Input: part model. Units: mm. Frame: model coordinates. A direction names the side the tool comes from. Give positions to 0.01 mm unless a question says otherwise; leave off trailing zeros. Loops run counter-clockwise (first coordinate to the right, second up) from the corner with the lowest first, then second, coordinate; pieces in that order, holes last. Notation, with made-up numbers: (3.25, -32.75) -> (44.25, -32.75) arc R27 cw to (44.25, -1.75) -> close; hole circle Ø7 at (30, -40). An arc over 180 degrees is marked (long way). Use CSV: the item, a comma, the result in double quotes.
```python
from build123d import *

# Parameters (mm, degrees)
BOX044_W                  = 180
BOX044_H                  = 123
BOX044_DEPTH              = 8
BOX045_W                  = 140
BOX045_H                  = 90
BOX045_DEPTH              = 40
CYLINDER019_R             = 15
CYLINDER019_DEPTH         = 10
CYLINDER020_R             = 15
CYLINDER020_DEPTH         = 24
BOX046_W                  = 75
BOX046_H                  = 13
BOX046_DEPTH              = 20
BOX047_W                  = 171
BOX047_H                  = 15
BOX047_DEPTH              = 10
FUSION013_ROLL_ANGLE      = -90
FUSION013_PLACEMENT_ANGLE = -180


with BuildPart() as cube039:
    # Box044 → Box044 (new body)
    with BuildSketch(Plane.XY):
        with Locations((90, 61.5)):
            Rectangle(BOX044_W, BOX044_H)
    extrude(amount=BOX044_DEPTH)


with BuildPart() as cube040:
    # Box045 → Box045 (new body)
    with BuildSketch(Plane(origin=(10, 15, 0), x_dir=(1, 0, 0), z_dir=(0, 0, 1))):
        with Locations((70, 45)):
            Rectangle(BOX045_W, BOX045_H)
    extrude(amount=BOX045_DEPTH)


with BuildPart() as cylinder019:
    # Cylinder019 → Cylinder019 (new body)
    with BuildSketch(Plane(origin=(30, 104, 24), x_dir=(1, 0, 0), z_dir=(0, 1, 0))):
        Circle(CYLINDER019_R)
    extrude(amount=CYLINDER019_DEPTH)


with BuildPart() as cylinder020:
    # Cylinder020 → Cylinder020 (new body)
    with BuildSketch(Plane(origin=(130, 104, 24), x_dir=(1, 0, 0), z_dir=(0, 1, 0))):
        Circle(CYLINDER020_R)
    extrude(amount=CYLINDER020_DEPTH)


with BuildPart() as cube041:
    # Box046 → Box046 (new body)
    with BuildSketch(Plane(origin=(193, 25, 0), x_dir=(0, 1, 0), z_dir=(0, 0, 1))):
        with Locations((37.5, 6.5)):
            Rectangle(BOX046_W, BOX046_H)
    extrude(amount=BOX046_DEPTH)


with BuildPart() as f_120_back:
    # Box047 → Box047 (new body)
    with BuildSketch(Plane(origin=(3, 0, 8), x_dir=(1, 0, 0), z_dir=(0, 0, 1))):
        with Locations((85.5, 7.5)):
            Rectangle(BOX047_W, BOX047_H)
    extrude(amount=BOX047_DEPTH)

    # Fusion013: union Cube039, Cube040, Cylinder019, Cylinder020, Cube041
    add(cube039.part)
    add(cube040.part)
    add(cylinder019.part)
    add(cylinder020.part)
    add(cube041.part)


with BuildPart() as f_120_back_1:
    # Fusion013 roll: moved
    add(f_120_back.part.rotate(Axis((0, 0, 0), (1, 0, 0)), FUSION013_ROLL_ANGLE))


with BuildPart() as f_120_back_2:
    # Fusion013 placement: moved
    add(f_120_back_1.part.moved(Location((195, -80, 185))).rotate(Axis((195, -80, 185), (0, 0, 1)), FUSION013_PLACEMENT_ANGLE))


solid = f_120_back_2.part
```
1) Ray query, line 1 (X direction, y = -95, z = 143); line 2 (X direction, y = -94, z = 177); line 3 (Z direction, x = 65, y = -101). Return the intervals inside material, ascending.
From the geometry:
line 1,"x = 2 to 15, 45 to 185"
line 2,"x = 21 to 192"
line 3,"z = 57 to 170"
2) Contact query for flat-ended pins moving along their axis: pin 1 (14.5 mm diameter, centred on x = 6.5, y = -93.5, fed in from +Z); pin 2 (8 mm diameter, centred on y = -94, z = 177, fed in from +X); pin 3 (15 mm diameter, centred on x = 163, y = -103, fed in from -Z). Output: stop coordinate, or through.
From the geometry:
pin 1,"stops at z = 160"
pin 2,"stops at x = 192"
pin 3,"stops at z = 71"
3) Reachability of faces 4 (the flat face through (192, -93, 178)), 5 (the flat face through (185, -104, 126)), 6 (the flat face through (108, -98, 177)) from +Z, -Z, +X, -X, +Y, -Y: full face, straight path, thin tool, end or side. Return the list, or none.
From the geometry:
face 4,"+Z, -Z, +X, -Y"
face 5,"-Z, +X, -Y"
face 6,"+Z, +X, -X, -Y"
4) Section query C-C (z = 138). Return loops of the section in (x, y).
From the geometry:
outline,"(2, -100) -> (15, -100) -> (15, -88) -> (45, -88) -> (45, -120) -> (185, -120) -> (185, -88) -> (195, -88) -> (195, -80) -> (2, -80) -> close"
5) Section query D-D (y = -104). Return loops of the section in (x, z), then the cut area to 3 significant figures.
From the geometry:
outline,"(45, 80) -> (50, 80) -> (50, 57) -> (80, 57) -> (80, 80) -> (150, 80) -> (150, 71) -> (180, 71) -> (180, 80) -> (185, 80) -> (185, 170) -> (45, 170) -> close"
area,"13,600 mm^2"
6) Mould query, pull axis Y, two halves, no side actions, for faces 1 (the flat face through (9, -100, 123)), 2 (the cylindrical face through (68.252, -118.643, 68.661)), 3 (the flat face through (2, -90, 123)). Classes: pulls with the +Y half, pulls with the -Y half, needs draft (parallel to the pull), parting line crosses it, or undercut.
From the geometry:
face 1,"pulls with the -Y half"
face 2,"undercut"
face 3,"needs draft"
7) Section query B-B (y = -95.5). Return loops of the section in (x, z).
From the geometry:
outline,"(2, 85) -> (15, 85) -> (15, 160) -> (2, 160) -> close; (21, 170) -> (45, 170) -> (45, 80) -> (52.64, 80) -> (52.64, 57) -> (77.36, 57) -> (77.36, 80) -> (152.64, 80) -> (152.64, 71) -> (177.36, 71) -> (177.36, 80) -> (185, 80) -> (185, 170) -> (192, 170) -> (192, 185) -> (21, 185) -> close"
8) Section query A-A (x = 165). Return loops of the section in (y, z), then the cut area to 3 significant figures.
From the geometry:
outline,"(-120, 80) -> (-119, 80) -> (-119, 71) -> (-89, 71) -> (-89, 80) -> (-88, 80) -> (-88, 62) -> (-80, 62) -> (-80, 185) -> (-98, 185) -> (-98, 170) -> (-120, 170) -> close"
area,"4,280 mm^2"
